from build123d import *

# Parameters (mm, degrees)
F0_W     = 140
F0_H     = 31.65
F1_DEPTH = 6.35
F2_W     = 140
F2_H     = 6.35
F3_DEPTH = 6.35
F4_R     = 4.33


with BuildPart() as f1:
    # F0 (on Top) → F1 (new body)
    with BuildSketch(Plane.XY):
        Rectangle(F0_W, F0_H)
    extrude(amount=F1_DEPTH)

    # F2 (on face) → F3 (join)
    with BuildSketch(Plane(origin=(0, 15.825, 0), x_dir=(-1, 0, 0), z_dir=(0, 1, 0))):
        with Locations((0, 3.175)):
            Rectangle(F2_W, F2_H)
        Polygon((-30, 86.35), (-70, 6.35), (70, 6.35), (30, 86.35), align=None)
    extrude(amount=F3_DEPTH)

    # F4
    f4_edges = [f1.edges().sort_by_distance(p)[0] for p in [
        (-70, -15.825, 3.175),
        (70, -15.825, 3.175),
        (70, 22.175, 3.175),
        (-70, 22.175, 3.175),
    ]]
    fillet(f4_edges, radius=F4_R)


solid = f1.part
The listing builds one solid part. Answer for the finished solid, in the listing's coordinates (mm). A direction names the side the tool comes from. Give positions to 0.01 mm unless a question says otherwise; leave off trailing zeros. Loops run counter-clockwise (first coordinate to the right, second up) from the corner with the lowest first, then second, coordinate; pieces in that order, holes last.
Item 1: A tool of negligible diameter and unlimited length cuts with its end or side. For faces 1 (the flat face through (1, 15.825, 38)), 2 (the flat face through (0, 19, 86.35)), from which of +Z, -Z, +X, -X, +Y, -Y can it reach the whole face along a straight path? Write none if from no direction.
Derived:
face 1: +Z, +X, -X, -Y
face 2: +Z, +X, -X, +Y, -Y
Item 2: A cutting plane is placed at D-D (z = 47). Give the vertices of the cut face in (x, y) (3 decimals).
Derived:
outline: (-49.675, 15.825) - (49.675, 15.825) - (49.675, 22.175) - (-49.675, 22.175) - close
Item 3: A cutting plane is placed at A-A (x = -42). Give the vertices of the cut face in (y, z) (3 decimals).
Derived:
outline: (-15.825, 0) - (22.175, 0) - (22.175, 62.35) - (15.825, 62.35) - (15.825, 6.35) - (-15.825, 6.35) - close
Item 4: A cutting plane is placed at C-C (x = 40). Give the vertices of the cut face in (y, z) (3 decimals).
Derived:
outline: (-15.825, 0) - (22.175, 0) - (22.175, 66.35) - (15.825, 66.35) - (15.825, 6.35) - (-15.825, 6.35) - close
Item 5: A cutting plane is placed at B-B (y = -3). Give the vertices of the cut face in (x, z).
Derived:
outline: (-70, 0) - (70, 0) - (70, 6.35) - (-70, 6.35) - close
Item 6: Find the intervals of material crossed by line 1 along Y through (x, z) = (-26, 49.5) (3 decimals); line 2 along Z through (x, y) = (-48, 6.5), in increasing order.
Derived:
line 1: y = 15.825 to 22.175
line 2: z = 0 to 6.35
Item 7: Each of these flat-tipped pins is pushed along its axis until it touches: pin 1 Ø1 at (x, z) = (-17, 46.5) entering from -Y (3 decimals); pin 2 Ø16 at (x, y) = (-19.5, -5.5) entering from +Z; pin 3 Ø8 at (y, z) = (17.5, 59) entering from +X (3 decimals). Where does it stop, or does it pass through?
Derived:
pin 1: stops at y = 15.825
pin 2: stops at z = 6.35
pin 3: stops at x = 45.675
